Input: dimensioned drawing with shaded views. Units: mm. Origin: part minimum x, y, z. A direction names the side the tool comes from. Give positions to 0.01 mm unless a question says otherwise; leave off trailing zeros. Write each loop counter-clockwise with the first axis right and the second up, starting at its lowest first coordinate (ties: lowest second). Pieces come first, ordered by that corner, then holes.
Q1. Section A-A (x = 12.5). Return the cut outline in (y, z).
Q2. Pin query (flat end, axial travel): pin 1 Ø7.5 at (y, z) = (8, 17) entering from +X; pin 2 Ø4.5 at (y, z) = (63, 6) entering from -X; pin 3 Ø8 at (y, z) = (44, 21) entering from +X; pin 4 Ø4.5 at (x, z) = (9, 7) entering from -Y. Return the tip coordinate at first contact, or that it passes through.
Q3. Section C-C (z = 19). Return the cut outline in (x, y).
Q4. Section B-B (y = 35). Return the cut outline in (x, z).
Q5. Mould query, pull axis Z, two halves, no side actions, for the marked faces 6, 7 and 8. Classes: +Z half, -Z half, draft (parallel to the pull), parting line (faces both ways), or undercut.
Q6. Line query: line 1 (Y direction, x = 1.1, z = 6); line 2 (Z direction, x = 10, y = 45); line 3 (Z direction, x = 16, y = 34). Output: solid intervals per line, ascending.
Q7. Section D-D (y = 7). Return the cut outline in (x, z), plus the area to 3 significant figures.
Q8. Reachability of the marked faces 1, 2, 3, 4 and 5 from +Z, -Z, +X, -X, +Y, -Y: full face, straight path, thin tool, end or side. Return the list, or none.
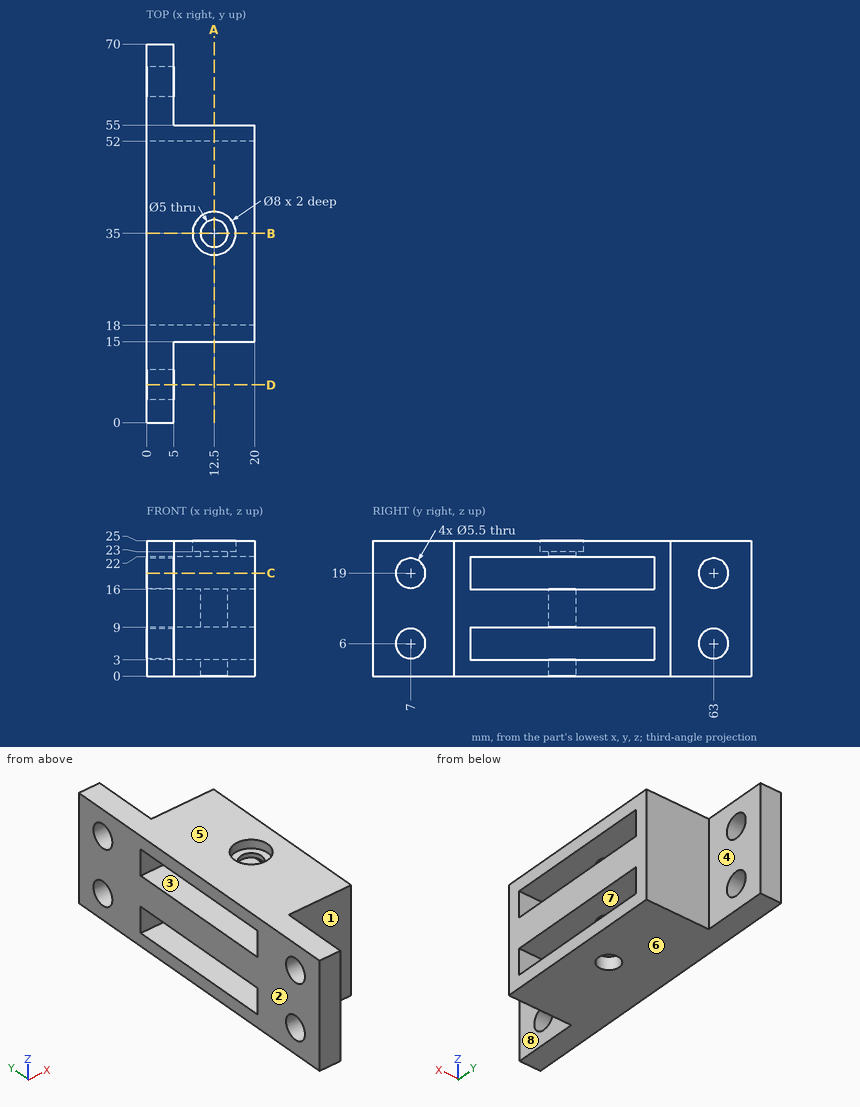
Computed:
1. outline: (15, 0) - (32.5, 0) - (32.5, 3) - (18, 3) - (18, 9) - (32.5, 9) - (32.5, 16) - (18, 16) - (18, 22) - (32.5, 22) - (32.5, 23) - (31, 23) - (31, 25) - (15, 25) - close; (37.5, 0) - (55, 0) - (55, 25) - (39, 25) - (39, 23) - (37.5, 23) - (37.5, 22) - (52, 22) - (52, 16) - (37.5, 16) - (37.5, 9) - (52, 9) - (52, 3) - (37.5, 3) - close
2. pin 1: stops at x = 5
2. pin 2: passes through
2. pin 3: stops at x = 20
2. pin 4: stops at y = 15
3. outline: (0, 0) - (5, 0) - (5, 4.25) - (0, 4.25) - close; (0, 9.75) - (5, 9.75) - (5, 15) - (20, 15) - (20, 18) - (0, 18) - close; (0, 52) - (20, 52) - (20, 55) - (5, 55) - (5, 60.25) - (0, 60.25) - close; (0, 65.75) - (5, 65.75) - (5, 70) - (0, 70) - close
4. outline: (0, 0) - (10, 0) - (10, 3) - (0, 3) - close; (0, 9) - (10, 9) - (10, 16) - (0, 16) - close; (0, 22) - (10, 22) - (10, 23) - (8.5, 23) - (8.5, 25) - (0, 25) - close; (15, 0) - (20, 0) - (20, 3) - (15, 3) - close; (15, 9) - (20, 9) - (20, 16) - (15, 16) - close; (15, 22) - (20, 22) - (20, 25) - (16.5, 25) - (16.5, 23) - (15, 23) - close
5. face 6: -Z half
5. face 7: undercut
5. face 8: draft
6. line 1: y = 0 to 4.25, 9.75 to 18, 52 to 60.25, 65.75 to 70
6. line 2: z = 0 to 3, 9 to 16, 22 to 25
6. line 3: z = 0 to 3, 9 to 16, 22 to 23
7. outline: (0, 0) - (5, 0) - (5, 3.25) - (0, 3.25) - close; (0, 8.75) - (5, 8.75) - (5, 16.25) - (0, 16.25) - close; (0, 21.75) - (5, 21.75) - (5, 25) - (0, 25) - close
7. area: 70.0 mm2
8. face 1: +Z, -Z, +X, -Y
8. face 2: +Z, -Z, -X, +Y, -Y
8. face 3: +X, -X
8. face 4: +Z, -Z, +X, +Y
8. face 5: +Z, +X, -X, +Y, -Y
